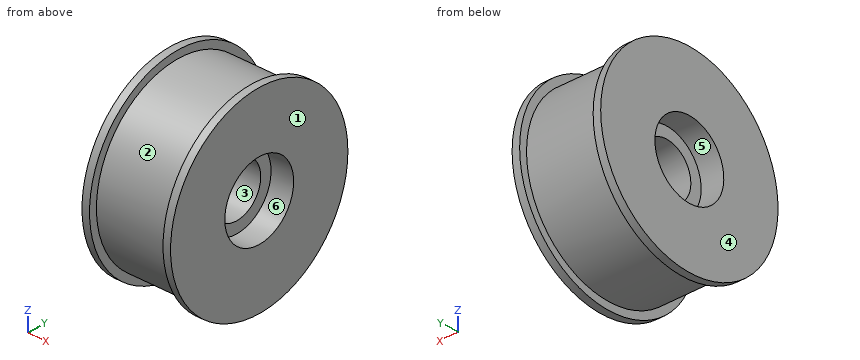
from build123d import *

# Parameters (mm, degrees)
SKETCH3_R          = 5
CUT_EXTRUDE1_DEPTH = 3
CUT_EXTRUDE2_START = -3
SKETCH4_R          = 5
CUT_EXTRUDE2_DEPTH = 3
SKETCH5_R          = 3.5
CUT_EXTRUDE3_DEPTH = 21.194957291


with BuildPart() as part:
    # Sketch2 → Revolve1 (revolve)
    with BuildSketch(Plane.XY):
        Polygon((0, 0), (0, 12.87), (1, 12.87), (1, 11.87), (10.75, 11.87), (10.75, 12.87), (11.75, 12.87), (11.75, 0), align=None)
    revolve(axis=Axis((11.75, 0, 0), (-1, 0, 0)))

    # Sketch3 → Cut-Extrude1 (cut)
    with BuildSketch(Plane(origin=(11.75, 0, 0), x_dir=(0, 0, -1), z_dir=(1, 0, 0))):
        Circle(SKETCH3_R)
    extrude(amount=-CUT_EXTRUDE1_DEPTH, mode=Mode.SUBTRACT)

    # Sketch4 → Cut-Extrude2 (cut)
    with BuildSketch(Plane.ZY.offset(CUT_EXTRUDE2_START)):
        with Locations(Location((0, 0, 0), (0, 0, 180))):
            Circle(SKETCH4_R)
    extrude(amount=CUT_EXTRUDE2_DEPTH, mode=Mode.SUBTRACT)

    # Sketch5 → Cut-Extrude3 (cut, through all)
    with BuildSketch(Plane(origin=(8.75, 0, 0), x_dir=(0, 0, -1), z_dir=(1, 0, 0))):
        Circle(SKETCH5_R)
    extrude(amount=-CUT_EXTRUDE3_DEPTH, mode=Mode.SUBTRACT)


solid = part.part
CAD build for the part. Positions are in the model's coordinates, mm. Face numbers are marked on the shaded views. A direction names the side the tool comes from. Round coordinates to 2 decimals unless told otherwise and drop trailing zeros. Write each loop counter-clockwise with the first axis right and the second up, starting at its lowest first coordinate (ties: lowest second). Pieces come first, ordered by that corner, then holes.
(1) Slice it at A-A, the plane y = 0. Write the cut outline in (x, z).
(2) Slice it at C-C, the plane x = 5.5. Write the cut outline in (y, z), and give its area (3 significant figures).
(3) Slice it at D-D, the plane y = 9. Write the cut outline in (x, z), and give its area (3 significant figures).
(4) 3-axis set-ups, long thin cutter, end or side, ignore diameter. For the marked faces 5 and 6: which of +Z, -Z, +X, -X, +Y, -Y reach the whole face in a straight line?
(5) Mould opens along X. For the marked faces 1, 2, 3 and 4 say: pulls with the +X half, pulls with the -X half, needs draft (parallel to the pull), parting line crosses it, or undercut.
(6) Drop flat-ended pins along their axis: P1, Ø4, axis at x = 9, y = -8.5, coming from the -Z side; P2, Ø1.5, axis at y = 0.5, z = -3.5, coming from the -X side; P3, Ø6, axis at y = 0, z = 0, coming from the +X side; P4, Ø2, axis at x = 8, y = -2, coming from the +Z side. Give the stop position or say it passes through.
(7) Probe line 1 along Y through (x, z) = (9.75, -0.25); line 2 along X through (y, z) = (10.75, -6.5); line 3 along Y through (x, z) = (6.25, 0). List the from-to ranges inside material, lowest first.
From the geometry:
1. outline: (0, -12.87) - (1, -12.87) - (1, -11.87) - (10.75, -11.87) - (10.75, -12.87) - (11.75, -12.87) - (11.75, -5) - (8.75, -5) - (8.75, -3.5) - (3, -3.5) - (3, -5) - (0, -5) - close; (0, 5) - (3, 5) - (3, 3.5) - (8.75, 3.5) - (8.75, 5) - (11.75, 5) - (11.75, 12.87) - (10.75, 12.87) - (10.75, 11.87) - (1, 11.87) - (1, 12.87) - (0, 12.87) - close
2. outline: circle Ø23.74 at (0, 0); hole circle Ø7 at (0, 0)
2. area: 404 mm2
3. outline: (0, -9.2) - (1, -9.2) - (1, -7.74) - (10.75, -7.74) - (10.75, -9.2) - (11.75, -9.2) - (11.75, 9.2) - (10.75, 9.2) - (10.75, 7.74) - (1, 7.74) - (1, 9.2) - (0, 9.2) - close
3. area: 188 mm2
4. face 5: -X
4. face 6: +X
5. face 1: pulls with the +X half
5. face 2: undercut
5. face 3: needs draft
5. face 4: pulls with the -X half
6. P1: stops at z = -10.44
6. P2: stops at x = 3
6. P3: passes through
6. P4: stops at z = 11.83
7. line 1: y = -11.87 to -4.99, 4.99 to 11.87
7. line 2: x = 0 to 1, 10.75 to 11.75
7. line 3: y = -11.87 to -3.5, 3.5 to 11.87
